Autodesk Inventor part; units mm, degrees
ref_plane "YZ Plane" through (0, 0, 0) normal (1, 0, 0) x (0, 1, 0)
ref_plane "XZ Plane" through (0, 0, 0) normal (0, 1, 0) x (-1, 0, 0)
ref_plane "XY Plane" through (0, 0, 0) normal (0, 0, 1) x (1, 0, 0)
sketch "Sketch1" plane through (0, 0, 0) normal (0, 0, 1) x (1, 0, 0)
  circle A0 centre (0, 0) radius 2.413
  circle A1 centre (0, 0) radius 6.35
  line L0 (1.3748, 2.3813) -> (2.7496, 0)
  line L1 (2.7496, 0) -> (1.3748, -2.3812)
  line L2 (1.3748, -2.3812) -> (-1.3748, -2.3812)
  line L3 (-1.3748, -2.3812) -> (-2.7496, 0)
  line L4 (-2.7496, 0) -> (-1.3748, 2.3813)
  line L5 (-1.3748, 2.3813) -> (1.3748, 2.3813)
  dimension "d0" = 4.826
  dimension "d1" = 12.7
  dimension "d2" = 4.7625
extrude "Extrusion1" add sketch "Sketch1" against normal blind 19.05 contours A0 L1 L2 L3 L4 L5 L0 | L0 A0 | A0 L1 | L5 A0 | A0 L2 | L4 A0 | A0 L3
extrude "Extrusion2" add sketch "Sketch1" along normal blind 3.175 contours L0 A0 | A0 L1 | L5 A0 | A0 L2 | L4 A0 | A0 L3 | A1
extrude "Extrusion3" add sketch "Sketch1" along normal blind 1.651 contours A0 L1 L2 L3 L4 L5 L0 | A0 L0 L1 | A0 L5 L0 | L1 L2 A0 | A0 L4 L5 | L2 L3 A0 | A0 L3 L4
thread "Thread1"
chamfer "Chamfer1" distance 0.3969 angle 45 1 edges at (-2.413, 0, -19.05)
fillet "Fillet1" radius 3.175 1 edges at (-6.35, 0, 3.175)
properties part number "10 32 bolt 0.75"
Model file for the job. Use its own axes, mm. A direction names the side the tool comes from. Round coordinates to 2 decimals unless told otherwise and drop trailing zeros. Order: outer loops, then holes, each group sorted by start corner. A loop starts at its lowest first (then second) coordinate and runs counter-clockwise, first axis right, second up.
(1) Drill centre lines: line 1 (Z direction, x = 1.25, y = -1.5); line 2 (Z direction, x = 2.75, y = 4.5); line 3 (Y direction, x = 2.25, z = 2.25). Where is each one in solid material? Low to high.
(2) 3-axis set-ups, long thin cutter, end or side, ignore diameter. For faces 1 (the face through (0, -2.381, 2)), 2 (the face through (2, -2, 3.175)), 3 (the face through (3, 0, 0)): which of +Z, -Z, +X, -X, +Y, -Y reach the whole face in a straight line?
(3) Band-saw the part on B-B (z = -9.5). List the corners of the cut face in (x, y).
(4) Pin check, flat tips, straight feed: pin 1 (1.4 mm diameter, centred on x = 0.5, y = -1, fed in from +Z); pin 2 (5 mm diameter, centred on x = 2.5, z = -17, fed in from +Y); pin 3 (3 mm diameter, centred on x = -4, y = 5, fed in from +Z). Stop position of each tip, or through.
(5) Pull direction X, two halves, no side cores. Call faces 4 (the face through (0, 0, -19.05)), 5 (the face through (-2.072, 1.174, 2.402)), 6 (the face through (-2.05, -1.21, 2.4)), 7 (the face through (-1.915, -1.468, -9.196)): released by +X, released by -X, zero draft, split by the parting line, or undercut.
Verdict:
1. line 1: z = -19.05 to 1.65
1. line 2: z = 0 to 2.38
1. line 3: y = -4.93 to -0.87, 0.87 to 4.93
2. face 1: +Z
2. face 2: +Z, +X, -X, +Y, -Y
2. face 3: -Z
3. outline: circle Ø4.83 at (0, 0)
4. pin 1: stops at z = 1.65
4. pin 2: stops at y = 2.41
4. pin 3: stops at z = 2.66
5. face 4: zero draft
5. face 5: undercut
5. face 6: undercut
5. face 7: split by the parting line
